from build123d import *

# Parameters (mm, degrees)
SKETCH_1_W             = 669.944195316
SKETCH_1_H             = 25
EXTRUDE_1_DEPTH        = 2000
EXTRUDE_2_DEPTH        = 1900
EXTRUDE_3_DEPTH        = 1900
CUT_EXTRUDE_1_REACH    = 2058.168
SKETCH_5_W             = 21.650635094
SKETCH_5_H             = 100
SKETCH_5_W_2           = 80.005810729
HOLE_WIZARD_M5_2_D     = 4.2
PATTERN_LINEAR_2_COUNT = 5
PATTERN_LINEAR_2_PITCH = 50


with BuildPart() as part:
    # 草图1 → 凸台-拉伸1 (new body)
    with BuildSketch(Plane(origin=(0, 0, 0), x_dir=(1, 0, 0), z_dir=(0, 1, 0))):
        with Locations((-40.027902342, 0)):
            Rectangle(SKETCH_1_W, SKETCH_1_H)
    extrude(amount=EXTRUDE_1_DEPTH)

    # 草图2 → 凸台-拉伸2 (add)
    with BuildSketch(Plane.XZ):
        Polygon((294.944195316, 12.5), (362.411238515, 12.5), (384.061873609, 0), (362.411238515, -12.5), (294.944195316, -12.5), align=None)
    extrude(amount=-EXTRUDE_2_DEPTH)

    # 草图3 → 凸台-拉伸3 (add)
    with BuildSketch(Plane.XZ):
        Polygon((-375, 12.5), (-455.005810729, 12.5), (-476.656445823, 0), (-455.005810729, -12.5), (-375, -12.5), align=None)
    extrude(amount=-EXTRUDE_3_DEPTH)

    # 草图5 → 切除-拉伸1 (cut, up to next)
    with BuildSketch(Plane(origin=(0, 0, -12.5), x_dir=(-1, 0, 0), z_dir=(0, 0, -1)), mode=Mode.PRIVATE) as cut_extrude_1_sk1:
        with Locations((465.831128276, 1250)):
            Rectangle(SKETCH_5_W, SKETCH_5_H)
    cut_extrude_1_tool1 = extrude(cut_extrude_1_sk1.sketch, amount=-CUT_EXTRUDE_1_REACH, mode=Mode.PRIVATE) & part.part
    # 草图5 → 切除-拉伸1 (cut, up to next)
    with BuildSketch(Plane(origin=(0, 0, -12.5), x_dir=(-1, 0, 0), z_dir=(0, 0, -1)), mode=Mode.PRIVATE) as cut_extrude_1_sk2:
        with Locations((415.002905365, 1250)):
            Rectangle(SKETCH_5_W_2, SKETCH_5_H)
    cut_extrude_1_tool2 = extrude(cut_extrude_1_sk2.sketch, amount=-CUT_EXTRUDE_1_REACH, mode=Mode.PRIVATE) & part.part
    add(cut_extrude_1_tool1.solids().sort_by_distance((-465.831128, 1250, -12.5))[0], mode=Mode.SUBTRACT)
    add(cut_extrude_1_tool2.solids().sort_by_distance((-415.002905, 1250, -12.5))[0], mode=Mode.SUBTRACT)

    # M5 螺纹孔2 (through all)
    with Locations(Plane(origin=(-341.225810729, 15, 12.5), x_dir=(1, 0, 0), z_dir=(0, 0, 1))):
        with Locations((0, 0)):
            hole_wizard_m5_2 = Hole(HOLE_WIZARD_M5_2_D / 2)

    # 阵列(线性)2: M5 螺纹孔2 ×5
    with Locations(*[(i * PATTERN_LINEAR_2_PITCH, 0, 0) for i in range(1, PATTERN_LINEAR_2_COUNT)]):
        add(hole_wizard_m5_2, mode=Mode.SUBTRACT)


solid = part.part
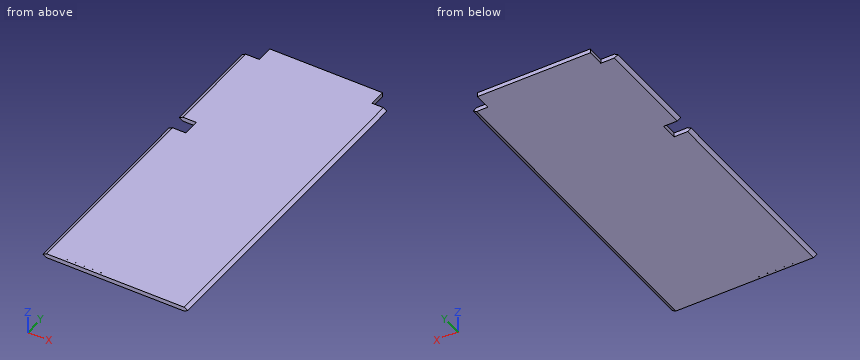
CAD build for the part. Positions are in the model's coordinates, mm. Round coordinates to 2 decimals unless told otherwise and drop trailing zeros. Order: outer loops, then holes, each group sorted by start corner. A loop starts at its lowest first (then second) coordinate and runs counter-clockwise, first axis right, second up. Notation, with made-up numbers: (23, 80.25) -> (61, 80.25) arc R23 cw to (61, 110.25) -> close; hole circle Ø4 at (-7, 38). An arc over 180 degrees is marked (long way). Write item = value, one per line. Start each with the question number.
(1) Cut at B-B, the plane y = 969. List the corners of the cut face in (x, z), then the cut area to 3 significant figures.
(2) Cut at A-A, the plane z = -5.5. List the corners of the cut face in (x, y).
(3) Cut at C-C, the plane x = 320. List the corners of the cut face in (y, z), then the cut area to 3 significant figures.
(4) Probe line 1 (Y direction, x = -379, z = 8.5); line 2 (X direction, y = 993, z = -5.25); line 3 (X direction, y = 1444, z = 0.5). List the from-to ranges inside material, lowest first. Write a range as [from, to].
(5) Pin check, flat tips, straight feed: P1, Ø1, axis at y = 434.5, z = -5.5, coming from the -X side; P2, Ø1, axis at x = 164.5, z = -8.5, coming from the -Y side; P3, Ø8, axis at y = 1659, z = 4.5, coming from the -X side; P4, Ø7.5, axis at y = 1965.5, z = 1.5, coming from the -X side. Stop position of each tip, or through.
Model answer:
q1.outline = (-476.66, 0) -> (-455.01, -12.5) -> (362.41, -12.5) -> (384.06, 0) -> (362.41, 12.5) -> (-455.01, 12.5) -> close
q1.area = 21,000 mm2
q2.outline = (-467.13, 0) -> (374.54, 0) -> (374.54, 1900) -> (294.94, 1900) -> (294.94, 2000) -> (-375, 2000) -> (-375, 1900) -> (-467.13, 1900) -> (-467.13, 1300) -> (-375, 1300) -> (-375, 1200) -> (-467.13, 1200) -> close; hole circle Ø4.2 at (-341.23, 15); hole circle Ø4.2 at (-291.23, 15); hole circle Ø4.2 at (-241.23, 15); hole circle Ø4.2 at (-191.23, 15); hole circle Ø4.2 at (-141.23, 15)
q3.outline = (0, -12.5) -> (1900, -12.5) -> (1900, 12.5) -> (0, 12.5) -> close
q3.area = 47,500 mm2
q4.line_1 = [0, 1200], [1300, 1900]
q4.line_2 = [-467.56, 374.97]
q4.line_3 = [-475.79, 383.2]
q5.P1 = -468
q5.P2 = 0
q5.P3 = -475.79
q5.P4 = -375
